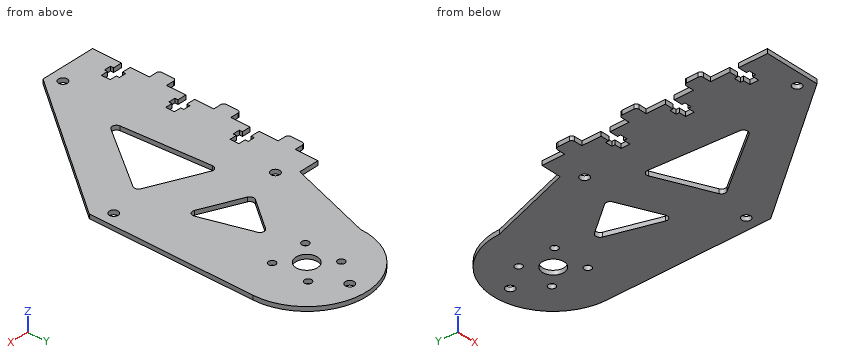
from build123d import *

# Parameters (mm, degrees)
SKETCH_1_R      = 5.0225
SKETCH_1_R_2    = 2.05
SKETCH_1_R_3    = 1.649999998
EXTRUDE_1_DEPTH = 2
FILLET_1_R      = 2
FILLET_2_R      = 1.3


with BuildPart() as part:
    # 草图1 → 凸台-拉伸1 (new body)
    with BuildSketch(Plane.XY):
        with BuildLine():
            Line((298.545628784, -83.894391363), (298.545628784, -92.841778663))
            Line((298.545628784, -92.841778663), (302.545628784, -92.841778663))
            Line((302.545628784, -92.841778663), (302.545628784, -91.391778663))
            Line((302.545628784, -91.391778663), (305.745628784, -91.391778663))
            Line((305.745628784, -91.391778663), (305.745628784, -92.841778663))
            Line((305.745628784, -92.841778663), (308.945628784, -92.841778663))
            Line((308.945628784, -92.841778663), (308.945628784, -96.941778663))
            Line((308.945628784, -96.941778663), (305.745628784, -96.941778663))
            Line((305.745628784, -96.941778663), (305.745628784, -98.391778663))
            Line((305.745628784, -98.391778663), (302.545628784, -98.391778663))
            Line((302.545628784, -98.391778663), (302.545628784, -96.941778663))
            Line((302.545628784, -96.941778663), (298.545628784, -96.941778663))
            Line((298.545628784, -96.941778663), (298.545628784, -105.894391358))
            Line((298.545628784, -105.894391358), (293.545628784, -105.894391358))
            Line((293.545628784, -105.894391358), (293.545628784, -113.894391358))
            Line((293.545628784, -113.894391358), (298.545628784, -113.894391358))
            Line((298.545628784, -113.894391358), (298.545628784, -122.847004054))
            Line((298.545628784, -122.847004054), (302.545628784, -122.847004054))
            Line((302.545628784, -122.847004054), (302.545628784, -121.397004054))
            Line((302.545628784, -121.397004054), (305.745628784, -121.397004054))
            Line((305.745628784, -121.397004054), (305.745628784, -122.847004054))
            Line((305.745628784, -122.847004054), (308.945628784, -122.847004054))
            Line((308.945628784, -122.847004054), (308.945628784, -126.947004054))
            Line((308.945628784, -126.947004054), (305.745628784, -126.947004054))
            Line((305.745628784, -126.947004054), (305.745628784, -128.397004054))
            Line((305.745628784, -128.397004054), (302.545628784, -128.397004054))
            Line((302.545628784, -128.397004054), (302.545628784, -126.947004054))
            Line((302.545628784, -126.947004054), (298.545628784, -126.947004054))
            Line((298.545628784, -126.947004054), (298.545628784, -140.447004054))
            Line((298.545628784, -140.447004054), (324.188862368, -140.447004054))
            Line((324.188862368, -140.447004054), (376.358604426, -71.946984141))
            Line((376.358604426, -71.946984141), (376.358604426, 4.396201153))
            ThreePointArc((376.358604426, 4.396201153), (348.536987634, 32.217817945), (320.715370843, 4.396201153))
            Line((320.715370843, 4.396201153), (307.936987634, -35.346984141))
            Line((307.936987634, -35.346984141), (298.545628784, -35.346984141))
            Line((298.545628784, -35.346984141), (298.545628784, -45.889165972))
            Line((298.545628784, -45.889165972), (293.545628784, -45.889165972))
            Line((293.545628784, -45.889165972), (293.545628784, -53.889165972))
            Line((293.545628784, -53.889165972), (298.545628784, -53.889165972))
            Line((298.545628784, -53.889165972), (298.545628784, -62.841778668))
            Line((298.545628784, -62.841778668), (302.545628784, -62.841778668))
            Line((302.545628784, -62.841778668), (302.545628784, -61.391778668))
            Line((302.545628784, -61.391778668), (305.745628784, -61.391778668))
            Line((305.745628784, -61.391778668), (305.745628784, -62.841778668))
            Line((305.745628784, -62.841778668), (308.945628784, -62.841778668))
            Line((308.945628784, -62.841778668), (308.945628784, -66.941778668))
            Line((308.945628784, -66.941778668), (305.745628784, -66.941778668))
            Line((305.745628784, -66.941778668), (305.745628784, -68.391778668))
            Line((305.745628784, -68.391778668), (302.545628784, -68.391778668))
            Line((302.545628784, -68.391778668), (302.545628784, -66.941778668))
            Line((302.545628784, -66.941778668), (298.545628784, -66.941778668))
            Line((298.545628784, -66.941778668), (298.545628784, -75.894391363))
            Line((298.545628784, -75.894391363), (293.545628784, -75.894391363))
            Line((293.545628784, -75.894391363), (293.545628784, -83.894391363))
            Line((293.545628784, -83.894391363), (298.545628784, -83.894391363))
        make_face()
        with Locations((348.536987634, 4.396201153)):
            Circle(SKETCH_1_R, mode=Mode.SUBTRACT)
        with Locations((348.537256281, 24.457337504)):
            Circle(SKETCH_1_R_2, mode=Mode.SUBTRACT)
        with Locations((320.545628784, -134.447004054)):
            Circle(SKETCH_1_R_2, mode=Mode.SUBTRACT)
        with Locations((370.358604426, -65.946984141)):
            Circle(SKETCH_1_R_2, mode=Mode.SUBTRACT)
        with Locations((313.936987634, -41.346984141)):
            Circle(SKETCH_1_R_2, mode=Mode.SUBTRACT)
        with Locations((340.172950793, 13.001018857)):
            Circle(SKETCH_1_R_3, mode=Mode.SUBTRACT)
        with Locations((357.141805339, 12.760237994)):
            Circle(SKETCH_1_R_3, mode=Mode.SUBTRACT)
        with Locations((356.901024475, -4.208616551)):
            Circle(SKETCH_1_R_3, mode=Mode.SUBTRACT)
        with Locations((339.93216993, -3.967835688)):
            Circle(SKETCH_1_R_3, mode=Mode.SUBTRACT)
        Polygon((354.947285032, -70.136765586), (328.579617375, -106.396108383), (325.08144343, -57.115165973), align=None, mode=Mode.SUBTRACT)
        Polygon((329.571126451, -37.254352656), (354.337315751, -48.052488042), (344.758747766, -17.175445836), align=None, mode=Mode.SUBTRACT)
    extrude(amount=EXTRUDE_1_DEPTH)

    # 圆角1
    fillet_1_edges = [part.edges().sort_by_distance(p)[0] for p in [
        (354.947285032, -70.136765586, 1),
        (325.08144343, -57.115165973, 1),
        (328.579617375, -106.396108383, 1),
        (344.758747766, -17.175445836, 1),
        (329.571126451, -37.254352656, 1),
        (354.337315751, -48.052488042, 1),
    ]]
    fillet(fillet_1_edges, radius=FILLET_1_R)

    # 圆角2
    fillet_2_edges = [part.edges().sort_by_distance(p)[0] for p in [
        (293.545628784, -113.894391358, 1),
        (293.545628784, -105.894391358, 1),
        (293.545628784, -83.894391363, 1),
        (293.545628784, -75.894391363, 1),
        (293.545628784, -53.889165972, 1),
        (293.545628784, -45.889165972, 1),
    ]]
    fillet(fillet_2_edges, radius=FILLET_2_R)


solid = part.part
Can you work these out from the model? Positions are in its coordinate system, mm. Give positions to 0.01 mm unless a question says otherwise; leave off trailing zeros. Order: outer loops, then holes, each group sorted by start corner. A loop starts at its lowest first (then second) coordinate and runs counter-clockwise, first axis right, second up. Notation, with made-up numbers: M 64,20 L 81,20 A10 cw 81,30 Z; hole C 81.5,11 d5. An arc over 180 degrees is marked long. Use one line per item in the form item = value. Start each with the question number.
Item 1: If we section it at B-B (x = 362.5): Write out the boundary of the cut face in (y, z), then the cut area to 3 significant figures.
Item 2: If we section it at A-A (z = 0.75): State how many separate pieces and enclosed holes the cut face has, then the cut area to 3 significant figures.
Item 3: If I drill on line 1 along Y through (x, z) = (300.5, 1.4); line 2 along Y through (x, z) = (344.5, 1.3); line 3 along Y through (x, z) = (331, 1.4), over which ranges is the centre line in solid material (lowest first)?
Item 4: Will these pins go through, and if not, where does the flat tip stop? pin 1 Ø12 at (x, y) = (356.5, -117.5) entering from -Z; pin 2 Ø0.6 at (x, z) = (307, 1) entering from +Y; pin 3 Ø1.2 at (y, z) = (-122.5, 1.5) entering from +X; pin 4 Ø2 at (x, y) = (348.5, -67.5) entering from +Z.
Item 5: If we section it at C-C (y = -9): Write out the boundary of the cut face in (x, z), then the cut area to 3 significant figures.
Outcome:
q1.outline = M -90.14,0 L 28.46,0 L 28.46,2 L -90.14,2 Z
q1.area = 237 mm2
q2.separate_pieces = 1
q2.enclosed_holes = 11
q2.area = 8,840 mm2
q3.line_1 = -140.45 to -126.95, -122.85 to -96.94, -92.84 to -66.94, -62.84 to -35.35
q3.line_2 = -113.78 to -84.5, -65.58 to -43.76, -19.55 to 1.41, 7.38 to 31.92
q3.line_3 = -131.5 to -102.61, -59.7 to -37.49, -35.38 to 25.99
q4.pin_1 = through
q4.pin_2 = -35.35
q4.pin_3 = 338.31
q4.pin_4 = 2
q5.outline = M 316.41,0 L 376.36,0 L 376.36,2 L 316.41,2 Z
q5.area = 120 mm2
